For this review, use the dimensioned drawing (mm, ordinates from the lowest corner) and the shaded views. A direction names the side the tool comes from. Round coordinates to 2 decimals unless told otherwise and drop trailing zeros. Loops run counter-clockwise (first coordinate to the right, second up) from the corner with the lowest first, then second, coordinate; pieces in that order, holes last. Notation, with made-up numbers: (55.25, 13.25) -> (102.25, 13.25) arc R20 ccw to (102.25, 22.25) -> close; hole circle Ø8 at (-21.75, 43.25). An arc over 180 degrees is marked (long way). Use one line per item in the form item = value. Start each with the question number.
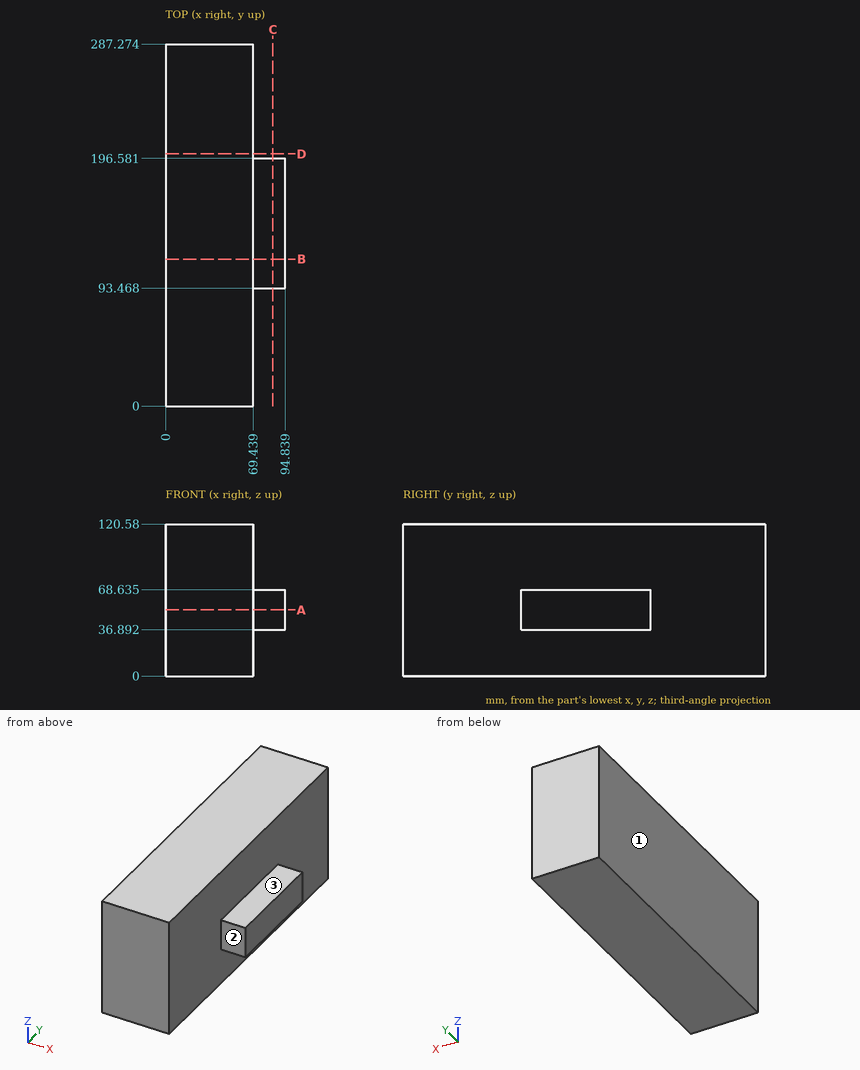
Item 1: Take a section at D-D on y = 200. Give the boundary of the cut face in (x, z), plus the area to 3 significant figures.
Item 2: Machinability: for the marked faces 1, 2 and 3, which of the approach directions +Z, -Z, +X, -X, +Y, -Y give a long, thin tool a straight path to every point of the face, cutting with its end or side? Answer none if there is none.
Item 3: Take a section at A-A on z = 52.5. Give the boundary of the cut face in (x, y), plus the area to 3 significant figures.
Item 4: Take a section at C-C on x = 85. Give the boundary of the cut face in (y, z) (1 decimal).
Item 5: Wall thickness on line 1 (X direction, y = 131, z = 10); line 2 (Z direction, x = 81.5, y = 139.5) (1 decimal): over which ranges is each line inside the solid? List them lowest first.
Item 6: For P1, Ø7.5, axis at x = 86, z = 45.5, coming from the -Y side; P2, Ø5, axis at y = 105, z = 93, coming from the +X side; P3, Ø7.5, axis at x = 81.5, y = 148.5, coming from the -Z side, all flat-tipped, find the tip position at first contact; note any pin that passes through.
Item 7: Take a section at B-B on y = 116.5. Give the boundary of the cut face in (x, z) (1 decimal), plus the area to 3 significant figures.
Results:
q1.outline = (0, 0) -> (69.44, 0) -> (69.44, 120.58) -> (0, 120.58) -> close
q1.area = 8,370 mm2
q2.face_1 = +Z, -Z, -X, +Y, -Y
q2.face_2 = +Z, -Z, +X, -Y
q2.face_3 = +Z, +X, +Y, -Y
q3.outline = (0, 0) -> (69.44, 0) -> (69.44, 93.47) -> (94.84, 93.47) -> (94.84, 196.58) -> (69.44, 196.58) -> (69.44, 287.27) -> (0, 287.27) -> close
q3.area = 22,600 mm2
q4.outline = (93.5, 36.9) -> (196.6, 36.9) -> (196.6, 68.6) -> (93.5, 68.6) -> close
q5.line_1 = 0 to 69.44
q5.line_2 = 36.9 to 68.6
q6.P1 = 93.47
q6.P2 = 69.44
q6.P3 = 36.89
q7.outline = (0, 0) -> (69.4, 0) -> (69.4, 36.9) -> (94.8, 36.9) -> (94.8, 68.6) -> (69.4, 68.6) -> (69.4, 120.6) -> (0, 120.6) -> close
q7.area = 9,180 mm2
